Here's how the part is built. I have some questions about the finished solid (model axes, mm). Round coordinates to 2 decimals unless told otherwise and drop trailing zeros. Write each loop counter-clockwise with the first axis right and the second up, starting at its lowest first coordinate (ties: lowest second). Pieces come first, ordered by that corner, then holes. Notation, with made-up numbers: M 48,-24.75 L 87,-24.75 A15 ccw 87,-15.75 Z; hole C 64.5,54.25 d10. An arc over 180 degrees is marked long. Use one line per item in the form item = value. Start each with the question number.
Q1. I want a section at A-A on z = 29. List the corners of the cut face in (x, y) for me.
Q2. I want a section at B-B on x = -130.5. List the corners of the cut face in (y, z) for me.
Q3. I need wall thicknesses on line 1 along X through (y, z) = (4, 9); line 2 along Z through (x, y) = (41.5, 6); line 3 along X through (y, z) = (6.5, 17). Which ranges of each line are inside material? Lowest first, please. Write a range as from..to.
Q4. I'm going to push flat-ended pins straight in: pin 1 Ø4 at (x, y) = (209.5, 7) entering from +Z; pin 2 Ø1.5 at (y, z) = (12.5, 20.5) entering from +X; pin 3 Ø4 at (y, z) = (12, 9.5) entering from +X. Where does each tip first touch, or does it pass through?
```python
from build123d import *

# Parameters (mm, degrees)
SKETCH1_W           = 100
SKETCH1_H           = 15
SKETCH1_R           = 5
BOSS_EXTRUDE1_DEPTH = 15
SKETCH1_2_R         = 5
BOSS_EXTRUDE2_DEPTH = 35
SKETCH2_R           = 0.4064
BOSS_EXTRUDE3_DEPTH = 420
BOSS_EXTRUDE4_START = -520
SKETCH2_2_R         = 0.4064
BOSS_EXTRUDE4_DEPTH = 520


with BuildPart() as part:
    # Sketch1 → Boss-Extrude1 (new body)
    with BuildSketch(Plane.XY):
        with Locations((50, 7.5)):
            Rectangle(SKETCH1_W, SKETCH1_H)
        with Locations((50, 7.5)):
            Circle(SKETCH1_R, mode=Mode.SUBTRACT)
    extrude(amount=BOSS_EXTRUDE1_DEPTH)

    # Sketch1_2 → Boss-Extrude2 (add)
    with BuildSketch(Plane.XY):
        with Locations((50, 7.5)):
            Circle(SKETCH1_2_R)
    extrude(amount=BOSS_EXTRUDE2_DEPTH)

    # Sketch2 → Boss-Extrude3 (add)
    with BuildSketch(Plane.ZY):
        with Locations(Location((7.5, 7.5, 0), (0, 0, 180))):
            Circle(SKETCH2_R)
    extrude(amount=BOSS_EXTRUDE3_DEPTH)

    # Sketch2_2 → Boss-Extrude4 (add)
    with BuildSketch(Plane.ZY.offset(BOSS_EXTRUDE4_START)):
        with Locations(Location((7.5, 7.5, 0), (0, 0, 180))):
            Circle(SKETCH2_2_R)
    extrude(amount=BOSS_EXTRUDE4_DEPTH)


solid = part.part
```
Reported:
q1.outline = C 50,7.5 d10
q2.outline = C 7.5,7.5 d0.81
q3.line_1 = 0..100
q3.line_2 = 0..15
q3.line_3 = 45.1..54.9
q4.pin_1 = 7.91
q4.pin_2 = 52.63
q4.pin_3 = 100
